from build123d import *

# Parameters (mm, degrees)
SKETCH1_R           = 250
BOSS_EXTRUDE1_DEPTH = 15
SKETCH2_R           = 30
BOSS_EXTRUDE2_DEPTH = 150
CIRPATTERN1_COUNT   = 3


with BuildPart() as part:
    # Sketch1 → Boss-Extrude1 (new body)
    with BuildSketch(Plane(origin=(0, 0, 0), x_dir=(1, 0, 0), z_dir=(0, 1, 0))):
        with Locations(Location((0, 0, 0), (0, 0, 270))):
            Circle(SKETCH1_R)
    extrude(amount=BOSS_EXTRUDE1_DEPTH)

    # Sketch2 → Boss-Extrude2 (add)
    with BuildSketch(Plane.XZ):
        with Locations(Location((200, 0, 0), (0, 0, 90))):
            Circle(SKETCH2_R)
    boss_extrude2 = extrude(amount=BOSS_EXTRUDE2_DEPTH)

    # CirPattern1: Boss-Extrude2 ×3 about axis
    cirpattern1_axis = Axis((0, 0, 0), (0, 1, 0))
    for i in range(1, CIRPATTERN1_COUNT):
        add(boss_extrude2.rotate(cirpattern1_axis, i * 360 / CIRPATTERN1_COUNT))


solid = part.part
Check sheet for the modelled part. Datum: model origin and axes. Units: mm. A direction names the side the tool comes from. Give positions to 0.01 mm unless a question says otherwise; leave off trailing zeros. Loops run counter-clockwise (first coordinate to the right, second up) from the corner with the lowest first, then second, coordinate; pieces in that order, holes last. Notation, with made-up numbers: M -36,-29.75 L 6,-29.75 A17 ccw 6,-24.75 Z; hole C -20,2 d3. An arc over 180 degrees is marked long. Use a Markdown table: item, result. Add a question column.
Q1. Sectioned sample at A-A, the plane x = 200. Record the cut outline in (y, z).
Q2. Sectioned sample at B-B, the plane z = 0. Record the cut outline in (x, y), then the cut area to 3 significant figures.
Q3. Sectioned sample at D-D, the plane x = -113. Record the cut outline in (y, z).
Q4. Go/stop test with flat-tipped pins: pin 1 (2 mm diameter, centred on y = -111, z = 185, fed in from +X); pin 2 (1 mm diameter, centred on x = -102, z = -98, fed in from -Y); pin 3 (8 mm diameter, centred on y = -48, z = 29.5, fed in from +X). Record where each tip stops, or that it passes through.
Q5. Scan lines: line 1 along Y through (x, z) = (157, -132); line 2 along Z through (x, y) = (-94, -122); line 3 along Z through (x, y) = (207, -74.5). Record each from-to range of solid material in increasing order. Write a range as [from, to].
Q6. Sectioned sample at C-C, the plane y = -138. Record the cut outline in (x, z).
Q7. Tool access check on faces 1 (the cylindrical face through (10.99, 7.4, -249.76)), 2 (the flat face through (4, 0, -3)). Record the directions out of +Z, -Z, +X, -X, +Y, -Y that give a thin tool (end or side, any length) a straight path to the whole face; none if there is none.
Verdict:
| question | item | result |
|---|---|---|
| 1 | outline | M -150,-30 L 0,-30 L 0,-150 L 15,-150 L 15,150 L 0,150 L 0,30 L -150,30 Z |
| 2 | outline | M -250,0 L 170,0 L 170,-150 L 230,-150 L 230,0 L 250,0 L 250,15 L -250,15 Z |
| 2 | area | 16,500 mm^2 |
| 3 | outline | M -150,-200.24 L 0,-200.24 L 0,-223 L 15,-223 L 15,223 L 0,223 L 0,200.24 L -150,200.24 L -150,146.17 L 0,146.17 L 0,-146.17 L -150,-146.17 Z |
| 4 | pin 1 | x = -72.01 |
| 4 | pin 2 | y = 0 |
| 4 | pin 3 | x = 215.8 |
| 5 | line 1 | [0, 15] |
| 5 | line 2 | [-202.6, -143.81], [143.81, 202.6] |
| 5 | line 3 | [-29.17, 29.17] |
| 6 | outline | C -100,-173.21 d60; C -100,173.21 d60; C 200,0 d60 |
| 7 | face 1 | +Y, -Y |
| 7 | face 2 | -Y |
